Answer from the drawing. Dimensions are ordinates in mm from the lowest x, y and z of the part. Give positions to 0.01 mm unless a question says otherwise; leave off trailing zeros. Order: outer loops, then holes, each group sorted by start corner. A loop starts at its lowest first (then second) coordinate and runs counter-clockwise, first axis right, second up. Notation, with made-up numbers: (37.5, -22.75) -> (53.5, -22.75) arc R24 ccw to (53.5, 10.25) -> close; hole circle Ø5 at (-8, -10). An arc over 180 degrees is marked (long way). One line per question, with ' | ' between items. Start each with the question number.
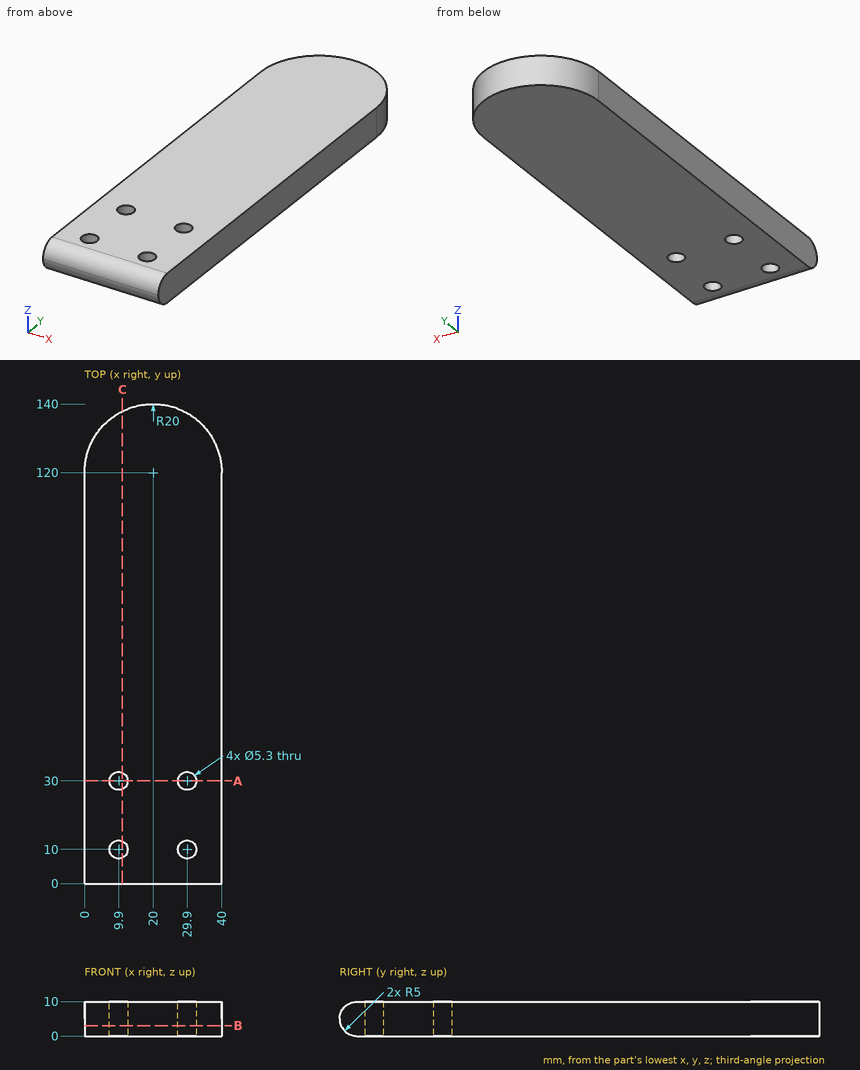
(1) The part is cut by section C-C on x = 11. State how many separate pieces and enclosed holes the cut face has, plus the area to 3 significant figures.
(2) Consider line 1 (Y direction, x = 9.9, z = 7.5); line 2 (Y direction, x = 9.9, z = 4.25); line 3 (Y direction, x = 38, z = 7.25) (1 decimal). Determine where each line is inside the solid, lowest interval first.
(3) The part is cut by section B-B on z = 3. Determine the outline of the cut face in (x, y).
(4) Given P1, Ø4, axis at x = 29.9, y = 30, coming from the -Z side; P2, Ø1.5, axis at x = 28.5, z = 8.5, coming from the -Y side; P3, Ø2, axis at x = 9, z = 3.5, coming from the +Y side, each flat-ended and moving along its own axis, determine where each tip first touches the part or whether it passes through.
(5) The part is cut by section A-A on y = 30. Determine the outline of the cut face in (x, z), plus the area to 3 significant figures.
Result sheet:
1) separate pieces: 3 | enclosed holes: 0 | area: 1,270 mm^2
2) line 1: y = 0.67 to 7.35, 12.65 to 27.35, 32.65 to 137.26 | line 2: y = 0.06 to 7.35, 12.65 to 27.35, 32.65 to 137.26 | line 3: y = 0.5 to 128.7
3) outline: (0, 0.42) -> (40, 0.42) -> (40, 120) arc R20 ccw to (0, 120) -> close; hole circle Ø5.3 at (9.9, 10); hole circle Ø5.3 at (9.9, 30); hole circle Ø5.3 at (29.9, 10); hole circle Ø5.3 at (29.9, 30)
4) P1: passes through | P2: stops at y = 0.82 | P3: stops at y = 137.32
5) outline: (0, 0) -> (7.25, 0) -> (7.25, 10) -> (0, 10) -> close; (12.55, 0) -> (27.25, 0) -> (27.25, 10) -> (12.55, 10) -> close; (32.55, 0) -> (40, 0) -> (40, 10) -> (32.55, 10) -> close | area: 294 mm^2
